from build123d import *

# Parameters (mm, degrees)
SKETCH_1_W          = 100
SKETCH_1_H          = 61
EXTRUDE_1_DEPTH     = 15
SKETCH_2_W          = 100
SKETCH_2_H          = 45
EXTRUDE_2_DEPTH     = 15
SKETCH_3_R          = 3.5
CUT_EXTRUDE_1_DEPTH = 121.917327129
SKETCH_4_R          = 5.5
CUT_EXTRUDE_2_DEPTH = 7
SKETCH_5_R          = 10
SKETCH_5_R_2        = 8
CUT_EXTRUDE_3_DEPTH = 121.917327129


with BuildPart() as part:
    # 草图1 → 凸台-拉伸1 (new body)
    with BuildSketch(Plane.XY):
        with Locations((50, 30.5)):
            Rectangle(SKETCH_1_W, SKETCH_1_H)
    extrude(amount=EXTRUDE_1_DEPTH)

    # 草图2 → 凸台-拉伸2 (add)
    with BuildSketch(Plane.XZ):
        with Locations((50, 7.5)):
            Rectangle(SKETCH_2_W, SKETCH_2_H)
    extrude(amount=EXTRUDE_2_DEPTH)

    # 草图3 → 切除-拉伸1 (cut, through all)
    with BuildSketch(Plane(origin=(0, 0, 0), x_dir=(1, 0, 0), z_dir=(0, 1, 0))):
        with Locations(Location((10, 7, 0), (0, 0, 270))):
            Circle(SKETCH_3_R)
        with Locations(Location((90, 7, 0), (0, 0, 270))):
            Circle(SKETCH_3_R)
        with Locations(Location((90, -22, 0), (0, 0, 90))):
            Circle(SKETCH_3_R)
        with Locations(Location((10, -22, 0), (0, 0, 90))):
            Circle(SKETCH_3_R)
    extrude(amount=-CUT_EXTRUDE_1_DEPTH, mode=Mode.SUBTRACT)

    # 草图4 → 切除-拉伸2 (cut)
    with BuildSketch(Plane(origin=(0, 0, 0), x_dir=(1, 0, 0), z_dir=(0, 1, 0))):
        with Locations(Location((10, 7, 0), (0, 0, 270))):
            Circle(SKETCH_4_R)
        with Locations(Location((90, 7, 0), (0, 0, 270))):
            Circle(SKETCH_4_R)
        with Locations(Location((10, -22, 0), (0, 0, 270))):
            Circle(SKETCH_4_R)
        with Locations(Location((90, -22, 0), (0, 0, 270))):
            Circle(SKETCH_4_R)
    extrude(amount=-CUT_EXTRUDE_2_DEPTH, mode=Mode.SUBTRACT)

    # 草图5 → 切除-拉伸3 (cut, through all)
    with BuildSketch(Plane(origin=(0, 0, 0), x_dir=(-1, 0, 0), z_dir=(0, 0, -1))):
        with Locations((-85, 46)):
            Circle(SKETCH_5_R)
        with Locations((-15, 46)):
            Circle(SKETCH_5_R)
        with Locations((-50, 46)):
            Circle(SKETCH_5_R_2)
    extrude(amount=-CUT_EXTRUDE_3_DEPTH, mode=Mode.SUBTRACT)


solid = part.part
Input: part model. Units: mm. Frame: model coordinates. A direction names the side the tool comes from. Round coordinates to 2 decimals unless told otherwise and drop trailing zeros. Write each loop counter-clockwise with the first axis right and the second up, starting at its lowest first coordinate (ties: lowest second). Pieces come first, ordered by that corner, then holes.
1) Contact query for flat-ended pins moving along their axis: P1, Ø1.5, axis at x = 42, y = 48, coming from the +Z side; P2, Ø16.5, axis at x = 27, z = -11, coming from the +Y side; P3, Ø23, axis at x = 15, y = 46, coming from the -Z side. Output: stop coordinate, or through.
2) Cut plane A-A (x = 21). Return the cut outline in (y, z), then the cut area to 3 significant figures.
3) Cut plane B-B (y = 46). Return the cut outline in (x, z).
4) Cut plane D-D (z = -7). Return the cut outline in (x, y).
5) Reachability of faces 1 (the cylindrical face through (93.417, -10.944, 22.759)), 2 (the cylindrical face through (95.453, -3.451, 21.284)), 3 (the flat face through (49, 0, -7)) from +Z, -Z, +X, -X, +Y, -Y: full face, straight path, thin tool, end or side. Return the list, or none.
6) Cut plane C-C (z = 6.5). Return the cut outline in (x, y), then the cut area to 3 significant figures.
7) Ray query, L1, parallel to X at y = -10, z = 22; L2, parallel to X at y = -5.5, z = 22; L3, parallel to Y at x = 14.5, z = 2. Return the intervals inside material, ascending.
8) Draft query along Z for faces 4 (the flat face through (49, 31, 0)), 5 (the cylindrical face through (51.041, 53.932, 7.395)), 6 (the cylindrical face through (86.583, -10.944, -7.759)). Return one class per face: pulls with the +Z half, pulls with the -Z half, needs draft (parallel to the pull), parting line crosses it, or undercut.
Geometry says:
1. P1: stops at z = 15
1. P2: stops at y = 0
1. P3: stops at z = 0
2. outline: (-15, -15) - (0, -15) - (0, 0) - (38, 0) - (38, 15) - (0, 15) - (0, 30) - (-15, 30) - close; (54, 0) - (61, 0) - (61, 15) - (54, 15) - close
2. area: 1,350 mm2
3. outline: (0, 0) - (5, 0) - (5, 15) - (0, 15) - close; (25, 0) - (42, 0) - (42, 15) - (25, 15) - close; (58, 0) - (75, 0) - (75, 15) - (58, 15) - close; (95, 0) - (100, 0) - (100, 15) - (95, 15) - close
4. outline: (0, -15) - (6.5, -15) - (6.5, -7) - (4.5, -7) - (4.5, 0) - (0, 0) - close; (13.5, -15) - (86.5, -15) - (86.5, -7) - (84.5, -7) - (84.5, 0) - (15.5, 0) - (15.5, -7) - (13.5, -7) - close; (93.5, -15) - (100, -15) - (100, 0) - (95.5, 0) - (95.5, -7) - (93.5, -7) - close
5. face 1: +Y, -Y
5. face 2: +Y
5. face 3: -Z, +X, -X, +Y
6. outline: (0, -15) - (100, -15) - (100, 61) - (0, 61) - close; hole circle Ø20 at (15, 46); hole circle Ø16 at (50, 46); hole circle Ø20 at (85, 46)
6. area: 6,770 mm2
7. L1: x = 0 to 6.5, 13.5 to 86.5, 93.5 to 100
7. L2: x = 0 to 4.5, 15.5 to 84.5, 95.5 to 100
7. L3: y = -15 to 36.01, 55.99 to 61
8. face 4: pulls with the -Z half
8. face 5: needs draft
8. face 6: undercut
